from build123d import *

# Parameters (mm, degrees)
F1_DEPTH = 3.175


with BuildPart() as f1:
    # F0 (on Right) → F1 (new body, symmetric)
    with BuildSketch(Plane.YZ):
        with BuildLine():
            Line((4.7625, 87.3125), (-4.7625, 87.3125))
            ThreePointArc((-4.7625, 87.3125), (-18.232884, 81.732884), (-23.8125, 68.2625))
            Line((-23.8125, 68.2625), (-23.8125, -80.9625))
            ThreePointArc((-23.8125, -80.9625), (-21.952628, -85.452628), (-17.4625, -87.3125))
            Line((-17.4625, -87.3125), (-3.175, -87.3125))
            Line((-3.175, -87.3125), (-3.175, -25.4))
            Line((-3.175, -25.4), (3.175, -25.4))
            Line((3.175, -25.4), (3.175, -87.3125))
            Line((3.175, -87.3125), (17.4625, -87.3125))
            ThreePointArc((17.4625, -87.3125), (21.952628, -85.452628), (23.8125, -80.9625))
            Line((23.8125, -80.9625), (23.8125, 68.2625))
            ThreePointArc((23.8125, 68.2625), (18.232884, 81.732884), (4.7625, 87.3125))
        make_face()
    extrude(amount=F1_DEPTH, both=True)


solid = f1.part
Work out the finished part from the listing and answer in its coordinate system (mm). A direction names the side the tool comes from. Give positions to 0.01 mm unless a question says otherwise; leave off trailing zeros. Loops run counter-clockwise (first coordinate to the right, second up) from the corner with the lowest first, then second, coordinate; pieces in that order, holes last. Notation, with made-up numbers: (89.5, 62.5) - (100.5, 62.5) arc R28 ccw to (100.5, 101.5) - close; hole circle Ø1 at (71, 28). An arc over 180 degrees is marked (long way). Answer in a Markdown table with one row per item. Add a question column.
Q1. The part is cut by section C-C (y = 1.5). Determine the outline of the cut face in (x, z) (1 decimal), and give its area (3 significant figures).
Q2. The part is cut by section A-A (z = -34.5). Determine the outline of the cut face in (x, y) (1 decimal).
Q3. This flat-tipped pin is pushed along its axis until it touches: P1, Ø5, axis at y = -3, z = -47.5, coming from the -X side (3 decimals). Where does it stop, or does it pass through?
Q4. A tool of negligible diameter and unlimited length cuts with its end or side. For faces 1 (the flat face through (0, 0, -25.4)), 2 (the flat face through (-3.175, 0, 1)), from which of +Z, -Z, +X, -X, +Y, -Y can it reach the whole face along a straight path? Write none if from no direction.
Q5. The part is cut by section D-D (y = 16). Determine the outline of the cut face in (x, z) (1 decimal), and give its area (3 significant figures).
Q6. Consider line 1 along Y through (x, z) = (0.5, -63) (1 decimal); line 2 along Z through (x, y) = (-0.25, 21); line 3 along Z through (x, y) = (1.75, -2.5). Determine where each line is inside the solid, lowest interval first.
Q7. Determine the mould class of faces 3 (the flat face through (0, 0, 87.312)), 4 (the flat face through (0, -3.175, -57)), 5 (the flat face through (0, 3.175, -56)), 6 (the cylindrical face through (0.044, 21.903, -85.502)) for opening direction Y: released by +Y, released by -Y, zero draft, split by the parting line, or undercut.
Solution:
| question | item | result |
|---|---|---|
| 1 | outline | (-3.2, -25.4) - (3.2, -25.4) - (3.2, 87.3) - (-3.2, 87.3) - close |
| 1 | area | 716 mm² |
| 2 | outline | (-3.2, -23.8) - (3.2, -23.8) - (3.2, -3.2) - (-3.2, -3.2) - close; (-3.2, 3.2) - (3.2, 3.2) - (3.2, 23.8) - (-3.2, 23.8) - close |
| 3 | P1 | stops at x = -3.175 |
| 4 | face 1 | -Z, +X, -X |
| 4 | face 2 | +Z, -Z, -X, +Y, -Y |
| 5 | outline | (-3.2, -87.3) - (3.2, -87.3) - (3.2, 83.6) - (-3.2, 83.6) - close |
| 5 | area | 1,090 mm² |
| 6 | line 1 | y = -23.8 to -3.2, 3.2 to 23.8 |
| 6 | line 2 | z = -86.24 to 78.22 |
| 6 | line 3 | z = -25.4 to 87.31 |
| 7 | face 3 | zero draft |
| 7 | face 4 | undercut |
| 7 | face 5 | undercut |
| 7 | face 6 | released by +Y |
